Input: part model. Units: mm. Frame: model coordinates. A direction names the side the tool comes from. Round coordinates to 2 decimals unless told otherwise and drop trailing zeros. Order: outer loops, then holes, each group sorted by start corner. A loop starts at its lowest first (then second) coordinate and runs counter-clockwise, first axis right, second up. Notation, with made-up numbers: (11.25, -30) -> (30.25, -30) arc R12 cw to (30.25, -13) -> close; hole circle Ø5 at (-32.75, -6). An arc over 180 degrees is marked (long way). Use a Markdown table: item, result.
from build123d import *

# Parameters (mm, degrees)
RESSALTO_EXTRUS_O1_DEPTH = 70
CORTE_EXTRUS_O1_REACH    = 112
ESBO_O2_R                = 3.1
FILETE1_SIZE             = 30
FILETE1_SIZE_2           = 45
ESBO_O3_R                = 3.75
RESSALTO_EXTRUS_O2_DEPTH = 8


with BuildPart() as part:
    # Esboço1 → Ressalto-extrusão1 (new body)
    with BuildSketch(Plane.XY):
        Polygon((0, 0), (0, 60), (-8, 60), (-8, 8), (-60, 8), (-60, 0), align=None)
    extrude(amount=RESSALTO_EXTRUS_O1_DEPTH)

    # Esboço2 → Corte-extrusão1 (cut, up to next)
    with BuildSketch(Plane(origin=(0, 0, 0), x_dir=(0, 0, -1), z_dir=(1, 0, 0)), mode=Mode.PRIVATE) as corte_extrus_o1_sk1:
        with Locations((-60, 45)):
            Circle(ESBO_O2_R)
    corte_extrus_o1_tool1 = extrude(corte_extrus_o1_sk1.sketch, amount=-CORTE_EXTRUS_O1_REACH, mode=Mode.PRIVATE) & part.part
    # Esboço2 → Corte-extrusão1 (cut, up to next)
    with BuildSketch(Plane(origin=(0, 0, 0), x_dir=(0, 0, -1), z_dir=(1, 0, 0)), mode=Mode.PRIVATE) as corte_extrus_o1_sk2:
        with Locations((-10, 45)):
            Circle(ESBO_O2_R)
    corte_extrus_o1_tool2 = extrude(corte_extrus_o1_sk2.sketch, amount=-CORTE_EXTRUS_O1_REACH, mode=Mode.PRIVATE) & part.part
    add(corte_extrus_o1_tool1.solids().sort_by_distance((0, 45, 60))[0], mode=Mode.SUBTRACT)
    add(corte_extrus_o1_tool2.solids().sort_by_distance((0, 45, 10))[0], mode=Mode.SUBTRACT)

    # Filete1
    # an asymmetric fillet: 45, 30 mm, written as the material it adds along each edge
    with BuildSketch(Plane(origin=(-8, 8, 0), x_dir=(0, 1, 0), z_dir=(0, 0, 1))) as filete1_piece_1:
        with BuildLine():
            Bezier((FILETE1_SIZE, 0), (0, 0), (0, FILETE1_SIZE_2), weights=[1, 0.707106781, 1])
            Line((0, FILETE1_SIZE_2), (0, 0))
            Line((0, 0), (FILETE1_SIZE, 0))
        make_face()
    extrude(amount=70)

    # Esboço3 → Ressalto-extrusão2 (add)
    with BuildSketch(Plane(origin=(0, 0, 0), x_dir=(0, 0, -1), z_dir=(1, 0, 0))):
        with BuildLine():
            Line((-50.499916272, 60), (-19.500083728, 60))
            ThreePointArc((-19.500083728, 60), (-24.794661769, 62.187990647), (-27.000043214, 67.475348435))
            ThreePointArc((-27.000043214, 67.475348435), (-35, 75.449053432), (-42.999956786, 67.475348435))
            ThreePointArc((-42.999956786, 67.475348435), (-45.205338231, 62.187990647), (-50.499916272, 60))
        make_face()
        with Locations((-35, 67.449053432)):
            Circle(ESBO_O3_R, mode=Mode.SUBTRACT)
    extrude(amount=-RESSALTO_EXTRUS_O2_DEPTH)


solid = part.part
1) Cut plane A-A on y = 69. Return loops of the section in (x, z).
Answer key:
| item | result |
|---|---|
| outline | (-8, 27.15) -> (0, 27.15) -> (0, 31.59) -> (-8, 31.59) -> close; (-8, 38.41) -> (0, 38.41) -> (0, 42.85) -> (-8, 42.85) -> close |
2) Cut plane B-B on x = -56. Return loops of the section in (y, z).
Answer key:
| item | result |
|---|---|
| outline | (0, 0) -> (8, 0) -> (8, 70) -> (0, 70) -> close |
3) Set-up query: faces 1 (the face through (-4, 60, 60)), 2 (the face through (-4, 60, 10)), 3 (the face through (-8, 53, 35)). Return all of +Z, -Z, +X, -X, +Y, -Y with unobstructed straight access to the full face (end or side cutting, diameter ignored); none if empty.
Answer key:
| item | result |
|---|---|
| face 1 | +Z, +X, -X, +Y |
| face 2 | -Z, +X, -X, +Y |
| face 3 | +Z, -Z, -X, +Y |
4) Cut plane C-C on y = 50. Return loops of the section in (x, z), and give its area (3 significant figures).
Answer key:
| item | result |
|---|---|
| outline | (-8, 0) -> (0, 0) -> (0, 70) -> (-8, 70) -> close |
| area | 560 mm^2 |
5) Draft query along Z for faces 4 (the face through (-3.944, 62.246, 45.147)), 5 (the face through (-3.944, 75.447, 34.824)), 6 (the face through (-3.94, 47.61, 58.33)). Return one class per face: released by +Z, released by -Z, zero draft, split by the parting line, or undercut.
Answer key:
| item | result |
|---|---|
| face 4 | released by +Z |
| face 5 | split by the parting line |
| face 6 | undercut |
6) Ray query, probe 1 along Y at (x, z) = (-3, 35); probe 2 along Y at (x, z) = (-3, 10); probe 3 along X at (y, z) = (56, 9.5). Return the intervals inside material, ascending.
Answer key:
| item | result |
|---|---|
| probe 1 | y = 0 to 63.7, 71.2 to 75.45 |
| probe 2 | y = 0 to 41.9, 48.1 to 60 |
| probe 3 | x = -8 to 0 |
7) Contact query for flat-ended pins moving along their axis: P1, Ø7, axis at y = 67.45, z = 35, coming from the -X side; P2, Ø1, axis at x = -54, z = 17, coming from the +Y side; P3, Ø6.5, axis at x = -2.5, z = 63, coming from the +Y side; P4, Ø10, axis at y = 45, z = 60, coming from the -X side. Output: stop coordinate, or through.
Answer key:
| item | result |
|---|---|
| P1 | passes through |
| P2 | stops at y = 8 |
| P3 | stops at y = 60 |
| P4 | stops at x = -8 |
